Geometry: see drawing. Coordinates: mm, zero at the bounding-box minimum. A direction names the side the tool comes from. Give positions to 0.01 mm unless a question says otherwise; leave off trailing zeros. Write each loop counter-clockwise with the first axis right and the second up, starting at its lowest first coordinate (ties: lowest second). Pieces come first, ordered by that corner, then holes. Notation, with made-up numbers: (4, 50) - (11, 50) arc R10 cw to (11, 61) - close; hole circle Ø5 at (9, 55). An arc over 180 degrees is marked (long way). Use a Markdown table: item, result. Add a question column.
1. Pin query (flat end, axial travel): pin 1 (3 mm diameter, centred on y = 18.5, z = 11.5, fed in from +X); pin 2 (3 mm diameter, centred on x = 13, y = 16, fed in from -Z); pin 3 (6 mm diameter, centred on x = 31.75, z = 28.35, fed in from +Y) (3 decimals); pin 4 (5 mm diameter, centred on y = 12.5, z = 27, fed in from +X). Return the tip coordinate at first contact, or that it passes through.
2. Material intervals for probe 1 along X at (y, z) = (6.35, 31); probe 2 along Z at (x, y) = (23.5, 9.75); probe 3 along X at (y, z) = (20, 6.5), sorted ascending.
3. Section query A-A, the plane y = 20. Count the separate pieces of the cut face and the enclosed holes in it.
4. Mould query, pull axis X, two halves, no side actions, for the marked faces 1, 2 and 3. Classes: released by +X, released by -X, zero draft, split by the parting line, or undercut.
5. Set-up query: the marked faces 4 and 5. Return all of +Z, -Z, +X, -X, +Y, -Y with unobstructed straight access to the full face (end or side cutting, diameter ignored); none if empty.
6. Section query C-C, the plane y = 14.5. Return loops of the section in (x, z).
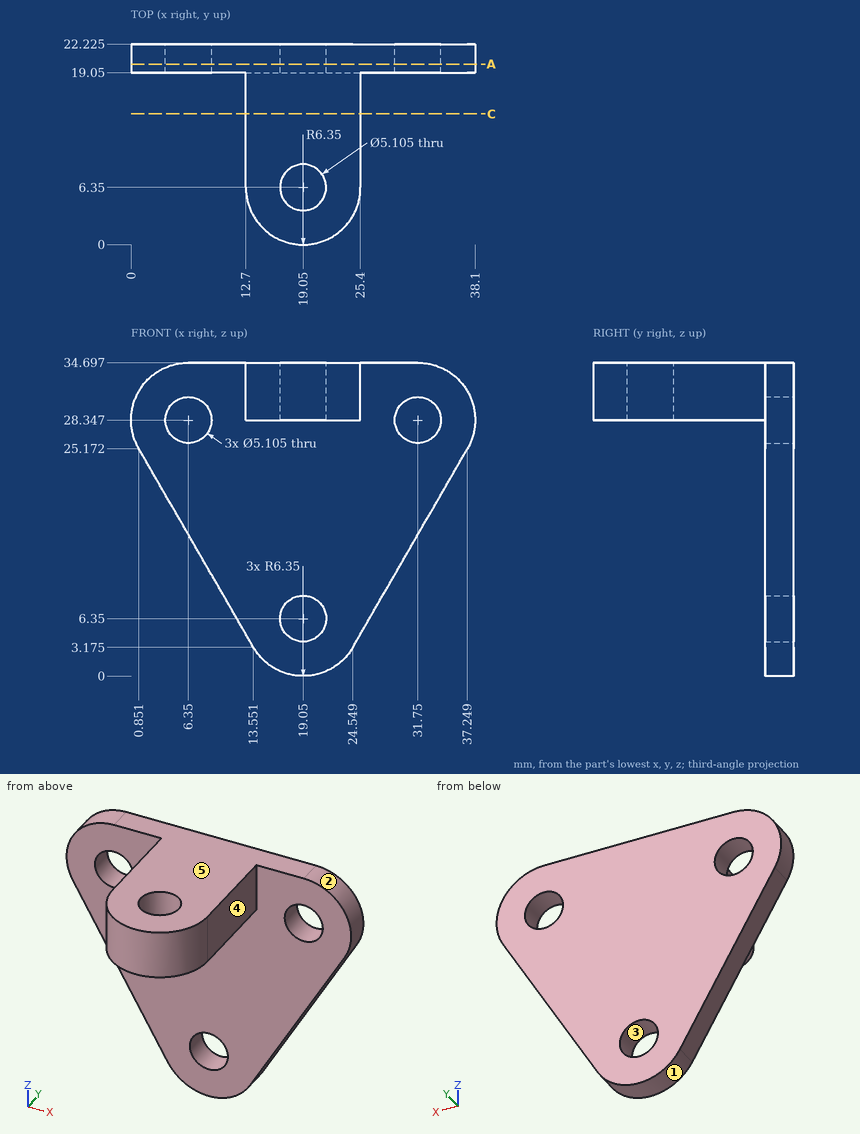
Result sheet:
| question | item | result |
|---|---|---|
| 1 | pin 1 | stops at x = 30.16 |
| 1 | pin 2 | stops at z = 28.35 |
| 1 | pin 3 | stops at y = 22.225 |
| 1 | pin 4 | stops at x = 25.4 |
| 2 | probe 1 | x = 12.7 to 16.5, 21.6 to 25.4 |
| 2 | probe 2 | z = 28.35 to 34.7 |
| 2 | probe 3 | x = 11.63 to 16.5, 21.6 to 26.47 |
| 3 | separate pieces | 1 |
| 3 | enclosed holes | 3 |
| 4 | face 1 | split by the parting line |
| 4 | face 2 | released by +X |
| 4 | face 3 | undercut |
| 5 | face 4 | +Z, -Z, +X, -Y |
| 5 | face 5 | +Z, +X, -X, +Y, -Y |
| 6 | outline | (12.7, 28.35) - (25.4, 28.35) - (25.4, 34.7) - (12.7, 34.7) - close |
